from build123d import *

# Parameters (mm, degrees)
F1_DEPTH = 5
F3_DEPTH = 4


with BuildPart() as f1:
    # F0 (on Top) → F1 (new body)
    with BuildSketch(Plane.XY):
        with BuildLine():
            Line((46.796926, 17.5), (55.296926, 17.5))
            ThreePointArc((55.296926, 17.5), (41.012193, 41.012193), (17.5, 55.296926))
            Line((17.5, 55.296926), (17.5, 46.796926))
            Line((17.5, 46.796926), (-17.5, 46.796926))
            Line((-17.5, 46.796926), (-17.5, 55.296926))
            ThreePointArc((-17.5, 55.296926), (-41.012193, 41.012193), (-55.296926, 17.5))
            Line((-55.296926, 17.5), (-46.796926, 17.5))
            Line((-46.796926, 17.5), (-46.796926, -17.5))
            Line((-46.796926, -17.5), (-55.296926, -17.5))
            ThreePointArc((-55.296926, -17.5), (-41.012193, -41.012193), (-17.5, -55.296926))
            Line((-17.5, -55.296926), (-17.5, -46.796926))
            Line((-17.5, -46.796926), (17.5, -46.796926))
            Line((17.5, -46.796926), (17.5, -55.296926))
            ThreePointArc((17.5, -55.296926), (41.012193, -41.012193), (55.296926, -17.5))
            Line((55.296926, -17.5), (46.796926, -17.5))
            Line((46.796926, -17.5), (46.796926, 17.5))
        make_face()
    extrude(amount=F1_DEPTH)

    # F2 (on face) → F3 (join)
    with BuildSketch(Plane.XY.offset(5)):
        Polygon((-28.921893, 34.50774), (-34.50774, 28.921893), (-17.377576, 11.791728), (-11.791728, 17.377576), align=None)
        Polygon((17.377576, 11.791728), (34.50774, 28.921893), (28.921893, 34.50774), (11.791728, 17.377576), align=None)
        Polygon((11.791728, -17.377576), (28.921893, -34.50774), (34.50774, -28.921893), (17.377576, -11.791728), align=None)
        Polygon((-17.377576, -11.791728), (-34.50774, -28.921893), (-28.921893, -34.50774), (-11.791728, -17.377576), align=None)
    extrude(amount=F3_DEPTH)


solid = f1.part
Could you check a few things on this model? Use its own coordinates, in mm. A direction names the side the tool comes from. Round coordinates to 2 decimals unless told otherwise and drop trailing zeros. Order: outer loops, then holes, each group sorted by start corner. A loop starts at its lowest first (then second) coordinate and runs counter-clockwise, first axis right, second up.
Q1. Which directions (+Z, -Z, +X, -X, +Y, -Y) give clear straight access to the entire face, cutting with the end or side of a thin tool? Please do faces 1 (the face through (0, -46.797, 2)), 2 (the face through (20.237, -25.823, 6.972)), 3 (the face through (25.823, 20.237, 6.972)), 4 (the face through (-1, 1, 5)), 5 (the face through (-25.823, -20.237, 6.972)).
Geometry says:
face 1: +Z, -Z, -Y
face 2: +Z, -Y
face 3: +Z, +X
face 4: +Z
face 5: +Z, -X
Q2. Imagine slicing it at C-C, the plane y = -32.5. List the corners of the cut face in (x, z) for me, then the cut area to 3 significant figures.
Geometry says:
outline: (-48.04, 0) - (48.04, 0) - (48.04, 5) - (30.93, 5) - (30.93, 9) - (26.91, 9) - (26.91, 5) - (-26.91, 5) - (-26.91, 9) - (-30.93, 9) - (-30.93, 5) - (-48.04, 5) - close
area: 513 mm2
Q3. Imagine slicing it at D-D, the plane z = 1.75. List the corners of the cut face in (x, y) for me.
Geometry says:
outline: (-55.3, -17.5) arc R58 ccw to (-17.5, -55.3) - (-17.5, -46.8) - (17.5, -46.8) - (17.5, -55.3) arc R58 ccw to (55.3, -17.5) - (46.8, -17.5) - (46.8, 17.5) - (55.3, 17.5) arc R58 ccw to (17.5, 55.3) - (17.5, 46.8) - (-17.5, 46.8) - (-17.5, 55.3) arc R58 ccw to (-55.3, 17.5) - (-46.8, 17.5) - (-46.8, -17.5) - close
Q4. I'm going to push flat-ended pins straight in: P1, Ø2, axis at y = -33.5, z = 3.5, coming from the +X side; P2, Ø4, axis at x = -52.5, z = 3, coming from the -Y side; P3, Ø1.5, axis at y = -49, z = 3.5, coming from the -X side. Where does each tip first touch, or does it pass through?
Geometry says:
P1: stops at x = 48.04
P2: stops at y = -28.53
P3: stops at x = -32.19
Q5. Thinking about a two-plate mould opening in Y: for faces 6 (the face through (-17.5, -51, 2)), 7 (the face through (46.797, 0, 2)), 8 (the face through (51, 17.5, 2)), 9 (the face through (31.75, 31.68, 6.97)), which applies, released by +Y, released by -Y, zero draft, split by the parting line, or undercut?
Geometry says:
face 6: zero draft
face 7: undercut
face 8: undercut
face 9: released by +Y
Q6. Please list where these lines run through material, in increasing order: probe 1 along Y at (x, z) = (14, 2.5); probe 2 along Z at (x, y) = (-23.5, -31); probe 3 along X at (y, z) = (19.5, 5.5).
Geometry says:
probe 1: y = -46.8 to 46.8
probe 2: z = 0 to 5
probe 3: x = -25.09 to -13.91, 13.91 to 25.09
Q7. Imagine slicing it at A-A, the plane z = 7.5. List the corners of the cut face in (x, y) for me, then the cut area to 3 significant figures.
Geometry says:
outline: (-34.51, -28.92) - (-28.92, -34.51) - (-11.79, -17.38) - (-17.38, -11.79) - close; (-34.51, 28.92) - (-17.38, 11.79) - (-11.79, 17.38) - (-28.92, 34.51) - close; (11.79, -17.38) - (28.92, -34.51) - (34.51, -28.92) - (17.38, -11.79) - close; (11.79, 17.38) - (17.38, 11.79) - (34.51, 28.92) - (28.92, 34.51) - close
area: 765 mm2
Q8. Imagine slicing it at B-B, the plane x = 32. List the corners of the cut face in (y, z) for me.
Geometry says:
outline: (-48.37, 0) - (48.37, 0) - (48.37, 5) - (31.43, 5) - (31.43, 9) - (26.41, 9) - (26.41, 5) - (-26.41, 5) - (-26.41, 9) - (-31.43, 9) - (-31.43, 5) - (-48.37, 5) - close
